Source: CAD feature listing. Evaluate the final solid. Frame: model axes, mm. A direction names the side the tool comes from. Coordinates: 2 decimals unless noted, no trailing zeros. Loops run counter-clockwise (first coordinate to the right, second up) from the corner with the lowest first, then second, coordinate; pieces in that order, holes last.
Item 1: Pin query (flat end, axial travel): pin 1 Ø12 at (x, y) = (39, 32) entering from -Z; pin 2 Ø6 at (y, z) = (49.5, 6.5) entering from -X; pin 3 Ø16 at (x, z) = (50.5, 13.5) entering from +Y; pin 4 Ø10 at (y, z) = (47, 11.5) entering from +X. Return the tip coordinate at first contact, or that it passes through.
Item 2: Reachability of faces 1 (the flat face through (118, 61, 10)), 2 (the flat face through (59, 4, 42)), 3 (the flat face through (59, 118, 10)), 4 (the cylindrical face through (4.406, 4.281, 9.86)), 5 (the flat face through (61, 2, 10)) from +Z, -Z, +X, -X, +Y, -Y: full face, straight path, thin tool, end or side. Return the list, or none.
Item 3: Section query B-B, the plane x = 85.5. Return the cut outline in (y, z).
Item 4: Section query A-A, the plane z = 52.5. Return the cut outline in (x, y).
Item 5: Line query: probe 1 along X at (y, z) = (16, 49); probe 2 along Y at (x, z) = (67.5, 17). Output: solid intervals per line, ascending.
Item 6: Pull-direction query (X, two-part tool) for faces 6 (the flat face through (116, 59, 42)), 7 (the cylindrical face through (115.594, 115.719, 9.86)), 8 (the cylindrical face through (5.711, 114.196, 43.602)), 9 (the flat face through (0, 59, 55)); classes: +X half, -X half, draft (parallel to the pull), parting line (faces both ways), or undercut.
```python
from build123d import *

# Parameters (mm, degrees)
SKETCH1_W           = 120
SKETCH1_H           = 120
BOSS_EXTRUDE1_DEPTH = 90
FILLET2_R           = 10
SHELL1_T            = -4
CUT_EXTRUDE1_DEPTH  = 20


with BuildPart() as part:
    # Sketch1 → Boss-Extrude1 (new body)
    with BuildSketch(Plane.XY):
        with Locations((60, 60)):
            Rectangle(SKETCH1_W, SKETCH1_H)
    extrude(amount=BOSS_EXTRUDE1_DEPTH)

    # Fillet2
    fillet2_edges = [part.edges().sort_by_distance(p)[0] for p in [
        (0, 0, 45),
        (120, 0, 45),
        (120, 120, 45),
        (0, 120, 45),
    ]]
    fillet(fillet2_edges, radius=FILLET2_R)

    # Shell1
    shell1_openings = [part.faces().sort_by_distance(p)[0] for p in [
        (60, 60, 0),
    ]]
    offset(amount=SHELL1_T, openings=shell1_openings, kind=Kind.INTERSECTION)

    # Sketch2 → Cut-Extrude1 (cut)
    with BuildSketch(Plane(origin=(0, 0, 0), x_dir=(-1, 0, 0), z_dir=(0, 0, -1))):
        with BuildLine():
            Line((-10, 120), (-110, 120))
            ThreePointArc((-110, 120), (-117.071067812, 117.071067812), (-120, 110))
            Line((-120, 110), (-120, 10))
            ThreePointArc((-120, 10), (-117.071067812, 2.928932188), (-110, 0))
            Line((-110, 0), (-10, 0))
            ThreePointArc((-10, 0), (-2.928932188, 2.928932188), (0, 10))
            Line((0, 10), (0, 110))
            ThreePointArc((0, 110), (-2.928932188, 117.071067812), (-10, 120))
        make_face()
        with BuildLine():
            Line((-10, 118), (-110, 118))
            ThreePointArc((-110, 118), (-115.656854249, 115.656854249), (-118, 110))
            Line((-118, 110), (-118, 10))
            ThreePointArc((-118, 10), (-115.656854249, 4.343145751), (-110, 2))
            Line((-110, 2), (-10, 2))
            ThreePointArc((-10, 2), (-4.343145751, 4.343145751), (-2, 10))
            Line((-2, 10), (-2, 110))
            ThreePointArc((-2, 110), (-4.343145751, 115.656854249), (-10, 118))
        make_face(mode=Mode.SUBTRACT)
    extrude(amount=-CUT_EXTRUDE1_DEPTH, mode=Mode.SUBTRACT)


solid = part.part
```
Verdict:
1. pin 1: stops at z = 86
1. pin 2: stops at x = 2
1. pin 3: stops at y = 120
1. pin 4: stops at x = 118
2. face 1: -Z, +X, +Y, -Y
2. face 2: -Z
2. face 3: -Z, +X, -X, +Y
2. face 4: -Z, -X, -Y
2. face 5: -Z, +X, -X, -Y
3. outline: (0, 20) - (2, 20) - (2, 0) - (4, 0) - (4, 86) - (116, 86) - (116, 0) - (118, 0) - (118, 20) - (120, 20) - (120, 90) - (0, 90) - close
4. outline: (0, 10) arc R10 ccw to (10, 0) - (110, 0) arc R10 ccw to (120, 10) - (120, 110) arc R10 ccw to (110, 120) - (10, 120) arc R10 ccw to (0, 110) - close; hole (4, 10) arc R6 ccw to (10, 4) - (110, 4) arc R6 ccw to (116, 10) - (116, 110) arc R6 ccw to (110, 116) - (10, 116) arc R6 ccw to (4, 110) - close
5. probe 1: x = 0 to 4, 116 to 120
5. probe 2: y = 2 to 4, 116 to 118
6. face 6: undercut
6. face 7: +X half
6. face 8: undercut
6. face 9: -X half
